Input: part model. Units: mm. Frame: model coordinates. Coordinates: 2 decimals unless noted, no trailing zeros. Order: outer loops, then holes, each group sorted by start corner. A loop starts at its lowest first (then second) coordinate and runs counter-clockwise, first axis right, second up. Notation, with made-up numbers: (14.5, 7) -> (25.5, 7) arc R16 ccw to (25.5, 32) -> close; hole circle Ø6 at (-26.5, -3.5). An arc over 180 degrees is marked (long way). Answer as CSV lines item,"result".
from build123d import *

# Parameters (mm, degrees)
F0_R     = 6.35
F1_DEPTH = 6.35


with BuildPart() as f1:
    # F0 (on Top) → F1 (new body)
    with BuildSketch(Plane.XY):
        with BuildLine():
            Line((-63.522818, 11.623597), (-63.522818, 24.323597))
            ThreePointArc((-63.522818, 24.323597), (-81.098645, 17.260726), (-88.9, 0))
            Line((-88.9, 0), (-71.09176, 6.765285))
            ThreePointArc((-71.09176, 6.765285), (-66.87415, 6.86833), (-63.522818, 4.30563))
            Line((-63.522818, 4.30563), (-63.522818, 11.623597))
        make_face()
        with BuildLine():
            ThreePointArc((-76.95588, -22.633602), (-70.508773, -25.496813), (-63.522818, -26.476403))
            Line((-63.522818, -26.476403), (-63.522818, -17.530432))
            Line((-63.522818, -17.530432), (-76.95588, -22.633602))
        make_face()
        with BuildLine():
            ThreePointArc((63.5, 0), (59.780256, 8.980256), (50.8, 12.7))
            Line((50.8, 12.7), (-39.801477, 12.7))
            ThreePointArc((-39.801477, 12.7), (-41.083686, 12.764892), (-42.35279, 12.958907))
            ThreePointArc((-42.35279, 12.958907), (-39.203292, 6.253034), (-38.122818, -1.076403))
            ThreePointArc((-38.122818, -1.076403), (-38.886391, -7.25754), (-41.1312, -13.067043))
            ThreePointArc((-41.1312, -13.067043), (-39.626671, -12.792095), (-38.1, -12.7))
            Line((-38.1, -12.7), (50.8, -12.7))
            ThreePointArc((50.8, -12.7), (59.780256, -8.980256), (63.5, 0))
        make_face()
        with Locations((50.661474, 0)):
            Circle(F0_R, mode=Mode.SUBTRACT)
        with BuildLine():
            ThreePointArc((-38.122818, -1.076403), (-39.203292, 6.253034), (-42.35279, 12.958907))
            ThreePointArc((-42.35279, 12.958907), (-44.282674, 13.516866), (-46.10043, 14.372163))
            Line((-46.10043, 14.372163), (-63.522818, 24.323597))
            Line((-63.522818, 24.323597), (-63.522818, 11.623597))
            Line((-63.522818, 11.623597), (-63.522818, 4.30563))
            ThreePointArc((-63.522818, 4.30563), (-63.178651, 3.711803), (-62.900585, 3.084299))
            Line((-62.900585, 3.084299), (-58.390395, -8.787861))
            ThreePointArc((-58.390395, -8.787861), (-58.53444, -13.645806), (-62.07138, -16.979036))
            Line((-62.07138, -16.979036), (-63.522818, -17.530432))
            Line((-63.522818, -17.530432), (-63.522818, -26.476403))
            Line((-63.522818, -26.476403), (-44.898486, -14.672904))
            ThreePointArc((-44.898486, -14.672904), (-43.079998, -13.717123), (-41.1312, -13.067043))
            ThreePointArc((-41.1312, -13.067043), (-38.886391, -7.25754), (-38.122818, -1.076403))
        make_face()
        with BuildLine():
            ThreePointArc((-46.10043, 14.372163), (-44.282674, 13.516866), (-42.35279, 12.958907))
            ThreePointArc((-42.35279, 12.958907), (-51.509011, 21.302793), (-63.522818, 24.323597))
            Line((-63.522818, 24.323597), (-46.10043, 14.372163))
        make_face()
        with BuildLine():
            ThreePointArc((-63.522818, -26.476403), (-50.472957, -22.867712), (-41.1312, -13.067043))
            ThreePointArc((-41.1312, -13.067043), (-43.079998, -13.717123), (-44.898486, -14.672904))
            Line((-44.898486, -14.672904), (-63.522818, -26.476403))
        make_face()
    extrude(amount=F1_DEPTH)


solid = f1.part
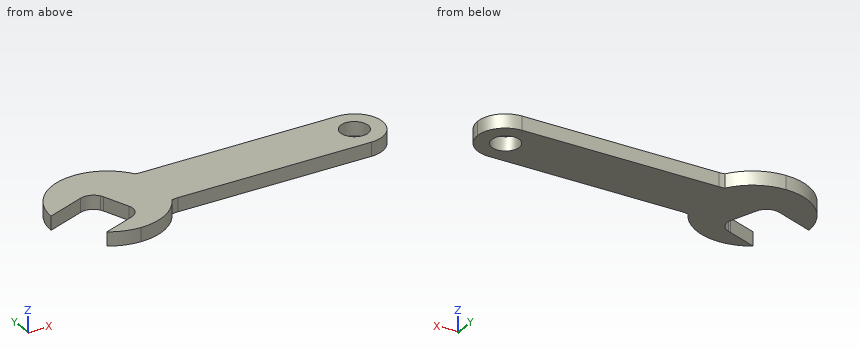
1. Cut plane B-B (x = 20). Return the cut outline in (y, z).
Findings:
outline,"(-12.7, 0) -> (12.7, 0) -> (12.7, 6.35) -> (-12.7, 6.35) -> close"
2. Ray query, line 1 along Y through (x, z) = (-12, 0.5); line 2 along Y through (x, z) = (-73, 2.5); line 3 along Y through (x, z) = (46, 3.5). Return the intervals inside material, ascending.
Findings:
line 1,"y = -12.7 to 12.7"
line 2,"y = -24.64 to -21.13, 6.04 to 22.49"
line 3,"y = -12.7 to -4.31, 4.31 to 12.7"
3. Contact query for flat-ended pins moving along their axis: pin 1 (10 mm diameter, centred on x = -46, y = -20, fed in from +Z); pin 2 (3 mm diameter, centred on x = 4.5, z = 5, fed in from +Y). Output: stop coordinate, or through.
Findings:
pin 1,"stops at z = 6.35"
pin 2,"stops at y = 12.7"
4. Cut plane A-A (z = 2). Return the cut outline in (x, y).
Findings:
outline,"(-88.9, 0) -> (-71.09, 6.77) arc R6.35 cw to (-63.52, 4.31) arc R6.35 cw to (-62.9, 3.08) -> (-58.39, -8.79) arc R6.35 cw to (-62.07, -16.98) -> (-76.96, -22.63) arc R25.4 ccw to (-63.52, -26.48) arc R25.4 ccw to (-41.13, -13.07) arc R12.7 cw to (-38.1, -12.7) -> (50.8, -12.7) arc R12.7 ccw to (50.8, 12.7) -> (-39.8, 12.7) arc R12.7 cw to (-42.35, 12.96) arc R25.4 ccw to (-63.52, 24.32) arc R25.4 ccw to start; hole circle Ø12.7 at (50.66, 0)"
5. Cut plane C-C (y = -19). Return the cut outline in (x, z).
Findings:
outline,"(-67.39, 0) -> (-45.53, 0) -> (-45.53, 6.35) -> (-67.39, 6.35) -> close"
